Build history of the part. All positions in model axes, mm. Give positions to 0.01 mm unless a question says otherwise; leave off trailing zeros. Order: outer loops, then holes, each group sorted by start corner. A loop starts at its lowest first (then second) coordinate and runs counter-clockwise, first axis right, second up. Notation, with made-up numbers: (12.25, 1.5) -> (65.25, 1.5) arc R23 ccw to (65.25, 29.5) -> close; hole circle Ø9 at (85.25, 80.5). An arc over 180 degrees is marked (long way). One line per item, written item: value. Start each with the question number.
(1) Saw through at A-A on z = 0. Give the cut face in (x, y), plus the area to 3 significant figures.
(2) Pin check, flat tip, straight feed: pin 1 (2.5 mm diameter, centred on y = 2, z = -17.5, fed in from +X). Stop position of the tip, or through.
(3) Two-plate mould, pull along X, no slides. Class faces 1 (the cylindrical face through (177.216, 2.576, -2.718)), 2 (the flat face through (-4, 5.08, -1)): +X half, -X half, draft (parallel to the pull), parting line (faces both ways), or undercut.
(4) Saw through at B-B on y = 4. Give the cut face in (x, z), plus the area to 3 significant figures.
(5) Probe line 1 (X direction, y = 2.05, z = 0); line 2 (X direction, y = 1.9, z = 11.5); line 3 (X direction, y = 0.2, z = 66). List the from-to ranges inside material, lowest first.
```python
from build123d import *

# Parameters (mm, degrees)
SKETCH1_W           = 635
SKETCH1_H           = 203.2
BOSS_EXTRUDE1_DEPTH = 5.08
SKETCH2_W           = 5.08
SKETCH2_H           = 25.4
SKETCH2_H_2         = 76.2
CUT_EXTRUDE1_DEPTH  = 5.08
SKETCH3_R           = 61.809841791
CUT_EXTRUDE2_DEPTH  = 5.08


with BuildPart() as part:
    # Sketch1 → Boss-Extrude1 (new body)
    with BuildSketch(Plane(origin=(0, 0, 0), x_dir=(1, 0, 0), z_dir=(0, 1, 0))):
        Rectangle(SKETCH1_W, SKETCH1_H)
    extrude(amount=BOSS_EXTRUDE1_DEPTH)

    # Sketch2 → Cut-Extrude1 (cut)
    with BuildSketch(Plane(origin=(0, 5.08, 0), x_dir=(1, 0, 0), z_dir=(0, 1, 0))):
        with Locations((314.96, 69.85)):
            Rectangle(SKETCH2_W, SKETCH2_H)
        with Locations((314.96, -69.85)):
            Rectangle(SKETCH2_W, SKETCH2_H)
        with Locations((314.96, 0)):
            Rectangle(SKETCH2_W, SKETCH2_H_2)
    extrude(amount=-CUT_EXTRUDE1_DEPTH, mode=Mode.SUBTRACT)

    # Sketch3 → Cut-Extrude2 (cut)
    with BuildSketch(Plane(origin=(0, 5.08, 0), x_dir=(1, 0, 0), z_dir=(0, 1, 0))):
        with Locations((238.966470336, 0)):
            Circle(SKETCH3_R)
    extrude(amount=-CUT_EXTRUDE2_DEPTH, mode=Mode.SUBTRACT)


solid = part.part
```
Results below:
1. outline: (-317.5, 0) -> (177.16, 0) -> (177.16, 5.08) -> (-317.5, 5.08) -> close; (300.78, 0) -> (312.42, 0) -> (312.42, 5.08) -> (300.78, 5.08) -> close
1. area: 2,570 mm²
2. pin 1: stops at x = 312.42
3. face 1: undercut
3. face 2: draft
4. outline: (-317.5, -101.6) -> (317.5, -101.6) -> (317.5, -82.55) -> (312.42, -82.55) -> (312.42, -57.15) -> (317.5, -57.15) -> (317.5, -38.1) -> (312.42, -38.1) -> (312.42, 38.1) -> (317.5, 38.1) -> (317.5, 57.15) -> (312.42, 57.15) -> (312.42, 82.55) -> (317.5, 82.55) -> (317.5, 101.6) -> (-317.5, 101.6) -> close; hole circle Ø123.62 at (238.97, 0)
4. area: 116,000 mm²
5. line 1: x = -317.5 to 177.16, 300.78 to 312.42
5. line 2: x = -317.5 to 178.24, 299.7 to 312.42
5. line 3: x = -317.5 to 312.42
